Read the model definition and answer for the solid it produces. Units are mm, in the model's axes. Face numbers are marked on the shaded views. Coordinates: 2 decimals unless noted, no trailing zeros. Write each loop counter-clockwise with the first axis right and the second up, starting at its lowest first coordinate (ties: lowest second). Pieces come first, ordered by that corner, then holes. Notation, with made-up numbers: M -10,17 L 5,17 A14 cw 5,26 Z; hole C 37.5,83.25 d11. An arc over 180 degrees is marked long. Write item = value, one per line.
from build123d import *

# Parameters (mm, degrees)
SKETCH1_R             = 25
SKETCH1_R_2           = 10
BOSS_EXTRUDE2_DEPTH   = 7
F_3_0MM_DOWEL_HOLE1_D = 3
CIRPATTERN1_COUNT     = 3


with BuildPart() as part:
    # Sketch1 → Boss-Extrude2 (new body)
    with BuildSketch(Plane.XY):
        Circle(SKETCH1_R)
        Circle(SKETCH1_R_2, mode=Mode.SUBTRACT)
    extrude(amount=BOSS_EXTRUDE2_DEPTH)

    # Ø3.0mm Dowel Hole1 (through all)
    with Locations(Plane.XY.offset(7)):
        with Locations((0, 21)):
            f_3_0mm_dowel_hole1 = Hole(F_3_0MM_DOWEL_HOLE1_D / 2)

    # CirPattern1: Ø3.0mm Dowel Hole1 ×3 about axis
    cirpattern1_axis = Axis((0, 0, 0), (0, 0, 1))
    for i in range(1, CIRPATTERN1_COUNT):
        add(f_3_0mm_dowel_hole1.rotate(cirpattern1_axis, i * 360 / CIRPATTERN1_COUNT), mode=Mode.SUBTRACT)


solid = part.part
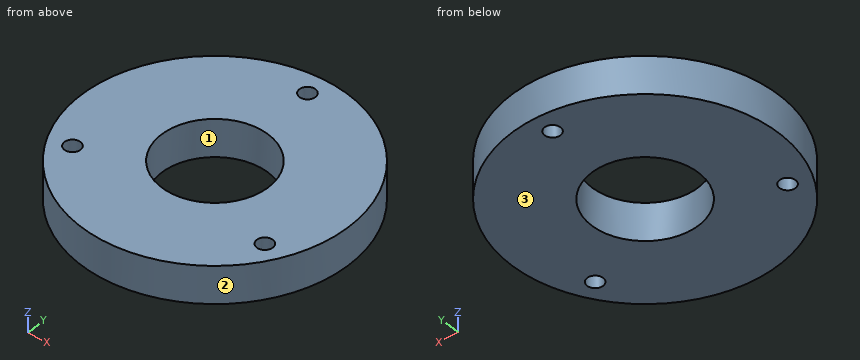
Item 1: For a pull along Y with two mould halves and no side action, classify the marked faces 1, 2 and 3 as released by +Y, released by -Y, zero draft, split by the parting line, or undercut.
Worked answers:
face_1 = undercut
face_2 = split by the parting line
face_3 = zero draft
Item 2: Find section C-C (x = -19). Determine the outline of the cut face in (y, z), and give its area (3 significant figures).
Worked answers:
outline = M -16.25,0 L -11.76,0 L -11.76,7 L -16.25,7 Z; M -9.24,0 L 16.25,0 L 16.25,7 L -9.24,7 Z
area = 210 mm²
Item 3: Consider line 1 along Y through (x, z) = (0, 4); line 2 along Y through (x, z) = (-5.5, 2.25); line 3 along Y through (x, z) = (-5, 4.75). Determine where each line is inside the solid, lowest interval first. Write a range as from..to.
Worked answers:
line_1 = -25..-10, 10..19.5, 22.5..25
line_2 = -24.39..-8.35, 8.35..24.39
line_3 = -24.49..-8.66, 8.66..24.49
Item 4: Find section B-B (x = 0). Determine the outline of the cut face in (y, z).
Worked answers:
outline = M -25,0 L -10,0 L -10,7 L -25,7 Z; M 10,0 L 19.5,0 L 19.5,7 L 10,7 Z; M 22.5,0 L 25,0 L 25,7 L 22.5,7 Z
Item 5: Find section A-A (y = 0). Determine the outline of the cut face in (x, z), and give its area (3 significant figures).
Worked answers:
outline = M -25,0 L -10,0 L -10,7 L -25,7 Z; M 10,0 L 25,0 L 25,7 L 10,7 Z
area = 210 mm²
Item 6: Flat-ended cylindrical pins translate along their axes: pin 1 (3 mm diameter, centred on y = 3.5, z = 1, fed in from +X); pin 2 (12 mm diameter, centred on x = -12.5, y = -18.5, fed in from -Z); pin 3 (1.8 mm diameter, centred on x = -18.19, y = -10.5, fed in from +Z); pin 4 (1.5 mm diameter, centred on y = -4, z = 3.5, fed in from +X). Find the tip coordinate at first contact, or state that the pin passes through.
Worked answers:
pin_1 = 24.92
pin_2 = 0
pin_3 = through
pin_4 = 24.79
Item 7: Find section D-D (z = 3.25). Determine the outline of the cut face in (x, y).
Worked answers:
outline = C 0,0 d50; hole C -18.19,-10.5 d3; hole C 0,0 d20; hole C 0,21 d3; hole C 18.19,-10.5 d3
